The listing builds one solid part. Answer for the finished solid, in the listing's coordinates (mm). Give positions to 0.01 mm unless a question says otherwise; leave off trailing zeros. Write each loop counter-clockwise with the first axis right and the second up, starting at its lowest first coordinate (ties: lowest second). Pieces come first, ordered by that corner, then holes. Notation, with made-up numbers: (36.5, 14) -> (75.5, 14) arc R24 ccw to (75.5, 51) -> close; hole circle Ø7 at (12.25, 75.5). An arc over 180 degrees is marked (long way). Put each result on its own line as item: value. Start each with the question number.
1) Flat-ended cylindrical pins translate along their axes: pin 1 Ø0.5 at (y, z) = (-0.5, -21) entering from +X (3 decimals); pin 2 Ø0.6 at (x, y) = (9.5, 0) entering from +Z (3 decimals); pin 3 Ø6 at (x, z) = (12.5, -15) entering from +Y. Find the tip coordinate at first contact, or state that the pin passes through.
2) Find the intervals of material crossed by line 1 along Z through (x, y) = (1.75, -0.4) (3 decimals); line 2 along X through (y, z) = (-0.4, -13) (3 decimals), in increasing order. Write a range as from..to.
3) A cutting plane is placed at A-A (y = -0.2). Write down the section's boundary in (x, z) (3 decimals).
4) A cutting plane is placed at B-B (x = 12). Write down the section's boundary in (y, z) (3 decimals), then the cut area to 3 significant figures.
5) A cutting plane is placed at C-C (z = 1.5). Write down the section's boundary in (x, y) (3 decimals), then the cut area to 3 significant figures.
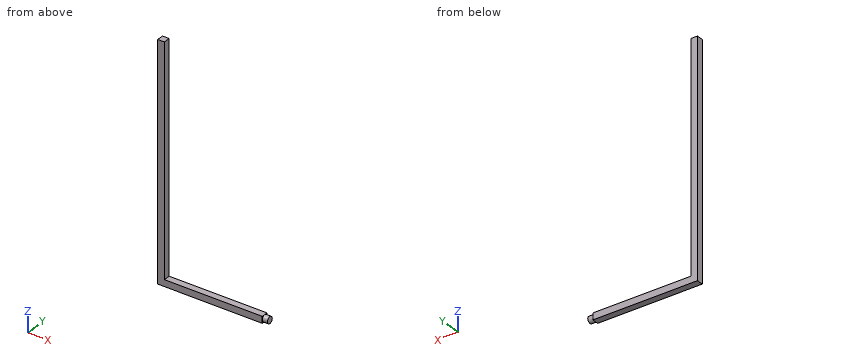
from build123d import *

# Parameters (mm, degrees)
SKETCH1_W           = 18.73
SKETCH1_H           = 1.27
SKETCH1_W_2         = 1.27
SKETCH1_H_2         = 43.18
BOSS_EXTRUDE1_DEPTH = 0.635
SKETCH2_R           = 0.635
BOSS_EXTRUDE2_DEPTH = 1


with BuildPart() as part:
    # Sketch1 → Boss-Extrude1 (new body, symmetric)
    with BuildSketch(Plane(origin=(0, 0, 0), x_dir=(1, 0, 0), z_dir=(0, 1, 0))):
        with Locations((10, 21.59)):
            Rectangle(SKETCH1_W, SKETCH1_H)
        with Locations((0, 21.59)):
            Rectangle(SKETCH1_W_2, SKETCH1_H)
        with Locations((0, -0.635)):
            Rectangle(SKETCH1_W_2, SKETCH1_H_2)
    extrude(amount=BOSS_EXTRUDE1_DEPTH, both=True)

    # Sketch2 → Boss-Extrude2 (add)
    with BuildSketch(Plane(origin=(19.365, 0, 0), x_dir=(0, 0, -1), z_dir=(1, 0, 0))):
        with Locations((21.59, 0)):
            Circle(SKETCH2_R)
    extrude(amount=BOSS_EXTRUDE2_DEPTH)


solid = part.part
Reply:
1. pin 1: stops at x = 20.365
1. pin 2: stops at z = -20.955
1. pin 3: passes through
2. line 1: z = -22.225..-20.955
2. line 2: x = -0.635..0.635
3. outline: (-0.635, -22.225) -> (19.365, -22.225) -> (19.365, -22.193) -> (20.365, -22.193) -> (20.365, -20.987) -> (19.365, -20.987) -> (19.365, -20.955) -> (0.635, -20.955) -> (0.635, 22.225) -> (-0.635, 22.225) -> close
4. outline: (-0.635, -22.225) -> (0.635, -22.225) -> (0.635, -20.955) -> (-0.635, -20.955) -> close
4. area: 1.61 mm2
5. outline: (-0.635, -0.635) -> (0.635, -0.635) -> (0.635, 0.635) -> (-0.635, 0.635) -> close
5. area: 1.61 mm2
